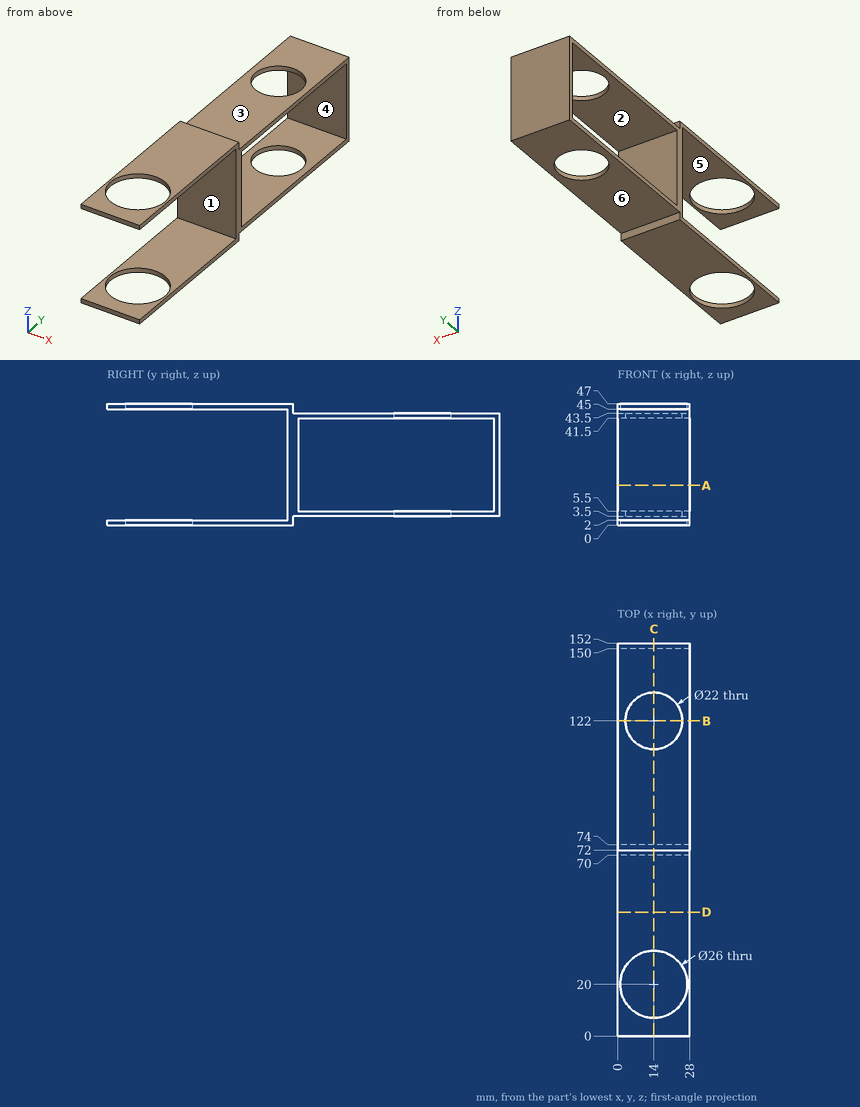
Input: dimensioned drawing with shaded views. Units: mm. Origin: part minimum x, y, z. A direction names the side the tool comes from. Give positions to 0.01 mm unless a question says otherwise; leave off trailing zeros. Write each loop counter-clockwise with the first axis right and the second up, starting at its lowest first coordinate (ties: lowest second). Pieces come first, ordered by that corner, then holes. Notation, with made-up numbers: (-31.75, 14.5) -> (-25.75, 14.5) arc R19 ccw to (-25.75, 38.5) -> close; hole circle Ø9 at (45.25, 83.5). An arc over 180 degrees is marked (long way). Answer as a JSON object with one key per item and string values.
1. Ray query, probe 1 along Z at (x, y) = (6.75, 86.5); probe 2 along Y at (x, z) = (12.75, 21.5); probe 3 along Y at (x, z) = (14, 46). Return the intervals inside material, ascending. Write a range as from..to.
Ans:
{"probe 1": "z = 3.5..5.5, 41.5..43.5", "probe 2": "y = 70..74, 150..152", "probe 3": "y = 0..7, 33..72"}
2. Access query for the marked faces 4, 5 and 6. Directions: +Z, -Z, +X, -X, +Y, -Y. A direction counts if a zero-diameter tool reaches every point of the face in a straight line with its end or side. Return the directions, or none.
Ans:
{"face 4": "+X, -X", "face 5": "+X, -X, -Y", "face 6": "-Z, +X, -X, +Y"}
3. Cut plane A-A on z = 15.5. Output: boundary loops of the cut face in (x, y).
Ans:
{"outline": "(0, 70) -> (28, 70) -> (28, 74) -> (0, 74) -> close; (0, 150) -> (28, 150) -> (28, 152) -> (0, 152) -> close"}
4. Cut plane D-D on y = 48. Output: boundary loops of the cut face in (x, z), and give its area (3 significant figures).
Ans:
{"outline": "(0, 0) -> (28, 0) -> (28, 2) -> (0, 2) -> close; (0, 45) -> (28, 45) -> (28, 47) -> (0, 47) -> close", "area": "112 mm^2"}
5. Cut plane C-C on x = 14. Count the separate pieces of the cut face and the enclosed holes in it, and give its area (3 significant figures).
Ans:
{"separate pieces": "4", "enclosed holes": "0", "area": "646 mm^2"}
6. Mould query, pull axis Y, two halves, no side actions, for the marked faces 1, 2 and 3. Classes: pulls with the +Y half, pulls with the -Y half, needs draft (parallel to the pull), parting line crosses it, or undercut.
Ans:
{"face 1": "pulls with the -Y half", "face 2": "undercut", "face 3": "needs draft"}
7. Cut plane B-B on y = 122. Output: boundary loops of the cut face in (x, z), and give its area (3 significant figures).
Ans:
{"outline": "(0, 3.5) -> (3, 3.5) -> (3, 5.5) -> (0, 5.5) -> close; (0, 41.5) -> (3, 41.5) -> (3, 43.5) -> (0, 43.5) -> close; (25, 3.5) -> (28, 3.5) -> (28, 5.5) -> (25, 5.5) -> close; (25, 41.5) -> (28, 41.5) -> (28, 43.5) -> (25, 43.5) -> close", "area": "24.0 mm^2"}
8. Contact query for flat-ended pins moving along their axis: pin 1 (14 mm diameter, centred on x = 12, z = 28, fed in from -Y); pin 2 (1 mm diameter, centred on x = 13, z = 2.5, fed in from +Y); pin 3 (1 mm diameter, centred on x = 24, y = 89.5, fed in from +Z). Output: stop coordinate, or through.
Ans:
{"pin 1": "stops at y = 70", "pin 2": "stops at y = 72", "pin 3": "stops at z = 43.5"}
